Input: dimensioned drawing with shaded views. Units: mm. Origin: part minimum x, y, z. A direction names the side the tool comes from. Give positions to 0.01 mm unless a question says otherwise; leave off trailing zeros. Write each loop counter-clockwise with the first axis right and the second up, starting at its lowest first coordinate (ties: lowest second). Pieces come first, ordered by that corner, then holes. Notation, with made-up numbers: (-39.5, -32.75) -> (13.5, -32.75) arc R18 cw to (13.5, -10.75) -> close; hole circle Ø4 at (27.25, 46). An arc over 180 degrees is marked (long way). Answer as a JSON object with one key per item and string values. Group by question number.
(1) Section query C-C on z = 1. Output: boundary loops of the cut face in (x, y).
(2) Contact query for flat-ended pins moving along their axis: pin 1 Ø3 at (x, y) = (7.5, 17) entering from +Z; pin 2 Ø2.5 at (x, y) = (16, 16) entering from -Z; pin 3 Ø2 at (x, z) = (7, 6.5) entering from -Y; pin 4 Ø2 at (x, z) = (24.5, 6.5) entering from +Y. Output: stop coordinate, or through.
(3) Set-up query: the marked faces 4 and 5. Return all of +Z, -Z, +X, -X, +Y, -Y with unobstructed straight access to the full face (end or side cutting, diameter ignored); none if empty.
(4) Section query A-A on y = 16. Output: boundary loops of the cut face in (x, z).
(5) Draft query along Y for the marked faces 1, 2 and 3. Return one class per face: +Y half, -Y half, draft (parallel to the pull), parting line (faces both ways), or undercut.
(6) Material intervals for probe 1 along Y at (x, z) = (16, 4.1); probe 2 along Y at (x, z) = (16, 7.6); probe 3 along Z at (x, y) = (2, 15), sorted ascending.
(7) Section query D-D on y = 12. Output: boundary loops of the cut face in (x, z).
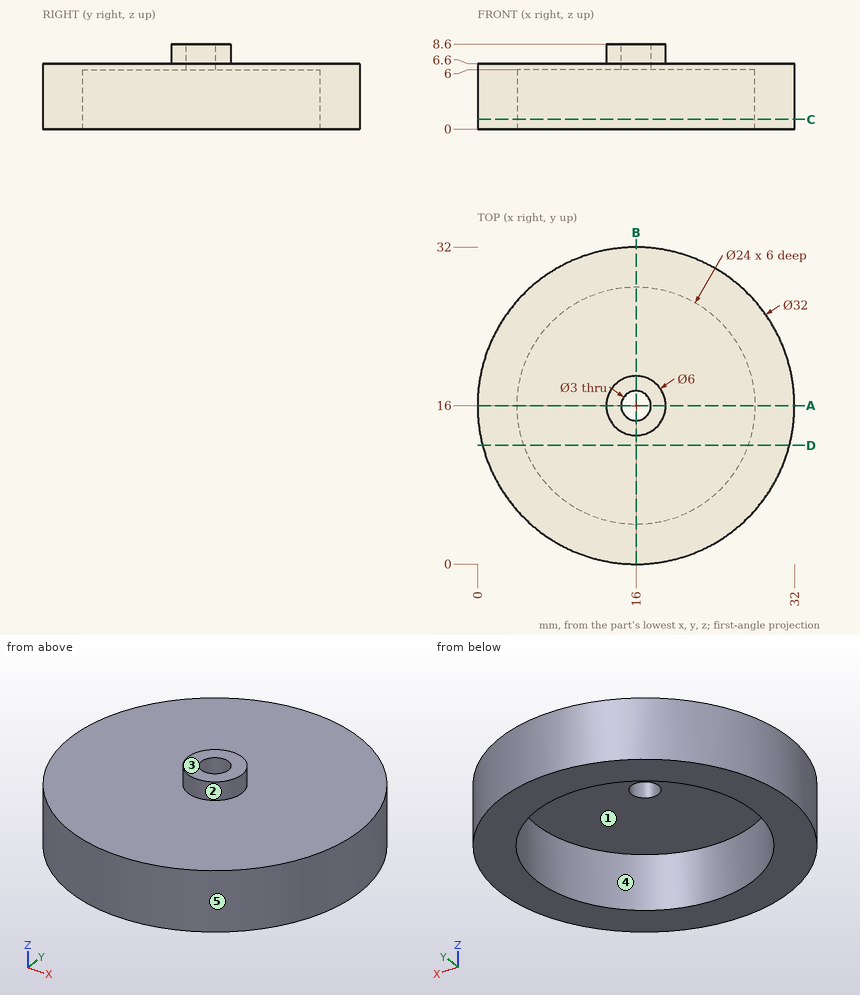
Answer list:
{
 "1": {"outline": "circle Ø32 at (16, 16); hole circle Ø24 at (16, 16)"},
 "2": {"pin 1": "z = 6.6", "pin 2": "through", "pin 3": "y = 2.14", "pin 4": "y = 30.13"},
 "3": {"face 4": "-Z", "face 5": "+Z, -Z"},
 "4": {"outline": "(0, 0) -> (4, 0) -> (4, 6) -> (14.5, 6) -> (14.5, 8.6) -> (13, 8.6) -> (13, 6.6) -> (0, 6.6) -> close; (17.5, 6) -> (28, 6) -> (28, 0) -> (32, 0) -> (32, 6.6) -> (19, 6.6) -> (19, 8.6) -> (17.5, 8.6) -> close"},
 "5": {"face 1": "undercut", "face 2": "parting line", "face 3": "draft"},
 "6": {"probe 1": "0 to 4, 28 to 32", "probe 2": "13 to 14.5, 17.5 to 19", "probe 3": "0 to 6.6"},
 "7": {"outline": "(0.51, 0) -> (4.69, 0) -> (4.69, 6) -> (27.31, 6) -> (27.31, 0) -> (31.49, 0) -> (31.49, 6.6) -> (0.51, 6.6) -> close"}
}
